Autodesk Inventor part; units mm, degrees
ref_plane "YZ Plane" through (0, 0, 0) normal (1, 0, 0) x (0, 1, 0)
ref_plane "XZ Plane" through (0, 0, 0) normal (0, 1, 0) x (-1, 0, 0)
ref_plane "XY Plane" through (0, 0, 0) normal (0, 0, 1) x (1, 0, 0)
sketch "スケッチ1" plane through (0, 0, 0) normal (0, 0, 1) x (1, 0, 0)
  line L0 (0, 0) -> (130, 0)
  line L1 (130, 0) -> (130, 40)
  line L2 (130, 40) -> (0, 40)
  line L3 (0, 40) -> (0, 0)
  dimension "d0" = 130
  dimension "d1" = 40
extrude "押し出し1" add sketch "スケッチ1" along normal blind 2
sketch "スケッチ2" plane through (0, 0, 2) normal (0, 0, 1) x (1, 0, 0)
  line L0 (130, 40) -> (0, 40)
  line L1 (0, 40) -> (130, 40)
  line L2 (130, 40) -> (130, 0)
  line L3 (130, 0) -> (0, 0)
  line L4 (0, 0) -> (0, 40)
  line L5 (7.5, 7.5) -> (122.5, 7.5)
  line L6 (122.5, 7.5) -> (122.5, 32.5)
  line L7 (122.5, 32.5) -> (7.5, 32.5)
  line L8 (7.5, 32.5) -> (7.5, 7.5)
  dimension "d4" = 7.5
extrude "押し出し2" cut sketch "スケッチ2" against normal blind 2 contours L8 L7 L6 L5
fillet "フィレット1" radius 2 8 edges at (0, 40, 1) (0, 0, 1) (7.5, 7.5, 1) (7.5, 32.5, 1) (130, 40, 1) (130, 0, 1) (122.5, 7.5, 1) (122.5, 32.5, 1)
properties part number "smaho_mount_board"
The listing builds one solid part. Answer for the finished solid, in the listing's coordinates (mm). Round coordinates to 2 decimals unless told otherwise and drop trailing zeros. Order: outer loops, then holes, each group sorted by start corner. A loop starts at its lowest first (then second) coordinate and runs counter-clockwise, first axis right, second up. Notation, with made-up numbers: (7.25, 15) -> (32.25, 15) arc R21 ccw to (32.25, 53) -> close; hole circle Ø1 at (1.5, 73.25). An arc over 180 degrees is marked (long way). Put each result on its own line as item: value.
Q1. Section C-C, the plane z = 1 is taken. Write down the section's boundary in (x, y).
Results list:
outline: (0, 2) arc R2 ccw to (2, 0) -> (128, 0) arc R2 ccw to (130, 2) -> (130, 38) arc R2 ccw to (128, 40) -> (2, 40) arc R2 ccw to (0, 38) -> close; hole (7.5, 9.5) arc R2 ccw to (9.5, 7.5) -> (120.5, 7.5) arc R2 ccw to (122.5, 9.5) -> (122.5, 30.5) arc R2 ccw to (120.5, 32.5) -> (9.5, 32.5) arc R2 ccw to (7.5, 30.5) -> close
Q2. Section A-A, the plane y = 24 is taken. Write down the section's boundary in (x, z), and give its area (3 significant figures).
Results list:
outline: (0, 0) -> (7.5, 0) -> (7.5, 2) -> (0, 2) -> close; (122.5, 0) -> (130, 0) -> (130, 2) -> (122.5, 2) -> close
area: 30.0 mm^2
Q3. Consider line 1 along Y through (x, z) = (55.5, 1.8); line 2 along X through (y, z) = (29, 0.65); line 3 along X through (y, z) = (31.5, 0.95). Determine where each line is inside the solid, lowest interval first.
Results list:
line 1: 0 to 7.5, 32.5 to 40
line 2: 0 to 7.5, 122.5 to 130
line 3: 0 to 7.77, 122.23 to 130
Q4. Section B-B, the plane x = 23 is taken. Write down the section's boundary in (y, z), and give its area (3 significant figures).
Results list:
outline: (0, 0) -> (7.5, 0) -> (7.5, 2) -> (0, 2) -> close; (32.5, 0) -> (40, 0) -> (40, 2) -> (32.5, 2) -> close
area: 30.0 mm^2
